Geometry: final body of the model. Coordinates: model frame, mm. Face numbers are marked on the shaded views. A direction names the side the tool comes from. Round coordinates to 2 decimals unless told otherwise and drop trailing zeros. Write each loop counter-clockwise with the first axis right and the second up, starting at its lowest first coordinate (ties: lowest second). Pieces come first, ordered by that corner, then holes. Notation, with made-up numbers: M 31,68 L 63,68 A33 ccw 63,105 Z; hole C -16,58.5 d6. An arc over 180 degrees is marked long. Answer as CSV lines item,"result". Start each with the question number.
Q1. Section query B-B on y = -7.5. Output: boundary loops of the cut face in (x, z).
Q2. Section query C-C on x = -4.5. Output: boundary loops of the cut face in (y, z).
Q3. Reachability of the marked faces 1, 2 and 3 from +Z, -Z, +X, -X, +Y, -Y: full face, straight path, thin tool, end or side. Return the list, or none.
Q4. Section query A-A on z = 9.5. Output: boundary loops of the cut face in (x, y).
Q5. First-contact query: pin 1 (3 mm diameter, centred on y = -14.5, z = 4, fed in from +X); pin 2 (5 mm diameter, centred on y = -13.5, z = 5.5, fed in from -X); pin 3 (5 mm diameter, centred on x = 35, y = -18.5, fed in from +Z). Flat tips, straight axial feed; report the tip coordinate or a pass-through.
Q6. Mould query, pull axis Z, two halves, no side actions, for the marked faces 4, 5 and 6. Classes: pulls with the +Z half, pulls with the -Z half, needs draft (parallel to the pull), parting line crosses it, or undercut.
Q7. Ray query, probe 1 along X at (y, z) = (-3.5, 9); probe 2 along Z at (x, y) = (10, -17); probe 3 along Z at (x, y) = (-35, -1.5). Return the intervals inside material, ascending.
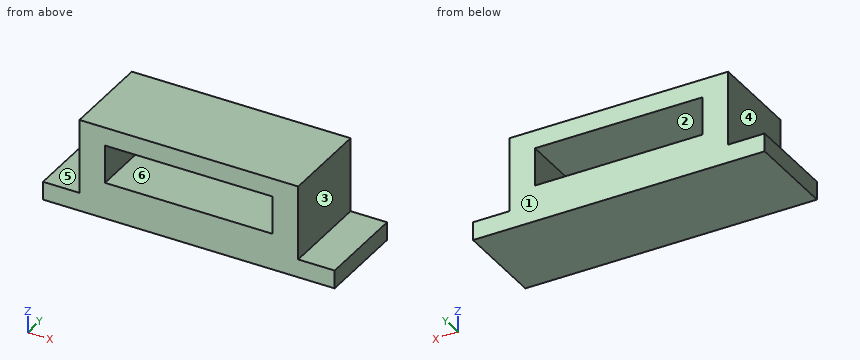
```python
from build123d import *

# Parameters (mm, degrees)
F0_W     = 60
F0_H     = 20.4615421835
F0_W_2   = 46
F0_H_2   = 10.4615421835
F1_DEPTH = 25


with BuildPart() as f1:
    # F0 (on Front) → F1 (new body)
    with BuildSketch(Plane.XZ):
        with Locations((-1.6490174871, 5.8380284264)):
            Rectangle(F0_W, F0_H)
        with Locations((-1.6490174871, 5.8380284264)):
            Rectangle(F0_W_2, F0_H_2, mode=Mode.SUBTRACT)
        Polygon((28.3509825129, -4.3927426653), (-31.6490174871, -4.3927426653), (-41.6490174871, -4.3927426653), (-41.6490174871, -9.3927426653), (38.3509825129, -9.3927426653), (38.3509825129, -4.3927426653), align=None)
    extrude(amount=F1_DEPTH)


solid = f1.part
```
Entries:
1,outline,"M -41.65,-9.39 L 38.35,-9.39 L 38.35,-4.39 L 28.35,-4.39 L 28.35,16.07 L -31.65,16.07 L -31.65,-4.39 L -41.65,-4.39 Z; hole M -24.65,0.61 L 21.35,0.61 L 21.35,11.07 L -24.65,11.07 Z"
2,outline,"M -25,-9.39 L 0,-9.39 L 0,0.61 L -25,0.61 Z; M -25,11.07 L 0,11.07 L 0,16.07 L -25,16.07 Z"
3,face 1,"+Z, -Z, +X, -X, +Y"
3,face 2,"+Y, -Y"
3,face 3,"+Z, +X, +Y, -Y"
4,outline,"M -31.65,-25 L -24.65,-25 L -24.65,0 L -31.65,0 Z; M 21.35,-25 L 28.35,-25 L 28.35,0 L 21.35,0 Z"
5,pin 1,"stops at x = 28.35"
5,pin 2,"stops at x = -31.65"
5,pin 3,"stops at z = -4.39"
6,face 4,"needs draft"
6,face 5,"pulls with the +Z half"
6,face 6,"undercut"
7,probe 1,"x = -31.65 to -24.65, 21.35 to 28.35"
7,probe 2,"z = -9.39 to 0.61, 11.07 to 16.07"
7,probe 3,"z = -9.39 to -4.39"
